Here's how the part is built. I have some questions about the finished solid (model axes, mm). Face numbers are marked on the shaded views. Round coordinates to 2 decimals unless told otherwise and drop trailing zeros. Loops run counter-clockwise (first coordinate to the right, second up) from the corner with the lowest first, then second, coordinate; pieces in that order, holes last. Notation, with made-up numbers: M 17,-21 L 51,-21 A19 cw 51,-11 Z; hole C 61,-5 d9. An arc over 180 degrees is marked long. Use a Markdown table: item, result.
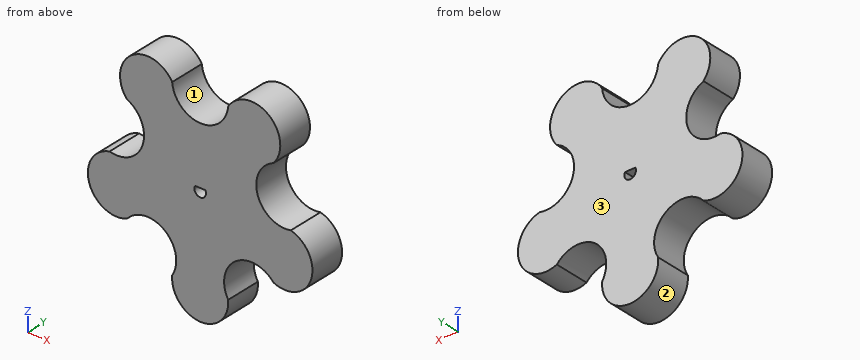
from build123d import *

# Parameters (mm, degrees)
BOSS_EXTRUDE1_DEPTH = 6.35
CUT_EXTRUDE1_DEPTH  = 87.982615074


with BuildPart() as part:
    # Sketch5 → Boss-Extrude1 (new body)
    with BuildSketch(Plane(origin=(0, 0, 0), x_dir=(1, 0, 0), z_dir=(0, 1, 0))):
        with BuildLine():
            ThreePointArc((63.790074828, 30.282665757), (58.727566665, 35.783867727), (53.665058502, 30.282665757))
            ThreePointArc((53.665058502, 30.282665757), (52.307776139, 23.537951339), (45.473748225, 24.331330481))
            ThreePointArc((45.473748225, 24.331330481), (38.677393188, 21.216564002), (42.344946112, 14.701867727))
            ThreePointArc((42.344946112, 14.701867727), (48.340127394, 11.326784114), (45.473748225, 5.072404972))
            ThreePointArc((45.473748225, 5.072404972), (46.335877976, -2.353828549), (53.665058502, -0.878930303))
            ThreePointArc((53.665058502, -0.878930303), (58.727566665, 3.779867727), (63.790074828, -0.878930303))
            ThreePointArc((63.790074828, -0.878930303), (71.119255353, -2.353828549), (71.981385104, 5.072404972))
            ThreePointArc((71.981385104, 5.072404972), (69.115005936, 11.326784114), (75.110187217, 14.701867727))
            ThreePointArc((75.110187217, 14.701867727), (78.777740141, 21.216564002), (71.981385104, 24.331330481))
            ThreePointArc((71.981385104, 24.331330481), (65.14735719, 23.537951339), (63.790074828, 30.282665757))
        make_face()
    extrude(amount=BOSS_EXTRUDE1_DEPTH)

    # Sketch6 → Cut-Extrude1 (cut, through all)
    with BuildSketch(Plane(origin=(0, 0, 0), x_dir=(1, 0, 0), z_dir=(0, 1, 0))):
        with BuildLine():
            Line((57.794311073, 14.225617727), (59.660822257, 14.225617727))
            ThreePointArc((59.660822257, 14.225617727), (58.727566665, 15.749617727), (57.794311073, 14.225617727))
        make_face()
    extrude(amount=CUT_EXTRUDE1_DEPTH, mode=Mode.SUBTRACT)


solid = part.part
1. Imagine slicing it at B-B, the plane x = 69.5. Write out the boundary of the cut face in (y, z).
Answer sheet:
| item | result |
|---|---|
| outline | M 0,-22.76 L 6.35,-22.76 L 6.35,-12.21 L 0,-12.21 Z; M 0,-7.3 L 6.35,-7.3 L 6.35,3.14 L 0,3.14 Z |
2. I need wall thicknesses on probe 1 along X at (y, z) = (5, -23.5); probe 2 along X at (y, z) = (2.5, -31); probe 3 along X at (y, z) = (2.25, -9.5). Which ranges of each line are inside material? Lowest first, please. Write a range as from..to.
Answer sheet:
| item | result |
|---|---|
| probe 1 | 40.2..46.39, 52.25..65.2, 71.07..77.26 |
| probe 2 | 53.66..63.8 |
| probe 3 | 48.58..68.87 |
3. Imagine slicing it at C-C, the plane y = 2.75. Write out the boundary of the cut face in (x, z).
Answer sheet:
| item | result |
|---|---|
| outline | M 42.34,-14.7 A5.08 ccw long 45.47,-24.33 A5.08 cw 53.67,-30.28 A5.08 ccw long 63.79,-30.28 A5.08 cw 71.98,-24.33 A5.08 ccw long 75.11,-14.7 A5.08 cw 71.98,-5.07 A5.08 ccw long 63.79,0.88 A5.08 cw 53.67,0.88 A5.08 ccw long 45.47,-5.07 A5.08 cw Z; hole M 57.79,-14.23 A1.05 ccw long 59.66,-14.23 Z |
4. For pin 1 Ø1.5 at (y, z) = (3.5, -22.5) entering from +X; pin 2 Ø1.5 at (x, y) = (66, 5.5) entering from -Z, each with a flat end and sliding along its axis, tell me the tip position at first contact or that it passes through.
Answer sheet:
| item | result |
|---|---|
| pin 1 | x = 78.57 |
| pin 2 | z = -23.47 |
5. Imagine slicing it at D-D, the plane z = -28. Write out the boundary of the cut face in (x, y).
Answer sheet:
| item | result |
|---|---|
| outline | M 54.39,0 L 63.07,0 L 63.07,6.35 L 54.39,6.35 Z |
6. Imagine slicing it at A-A, the plane z = -3. Write out the boundary of the cut face in (x, y).
Answer sheet:
| item | result |
|---|---|
| outline | M 44.4,0 L 56.02,0 L 56.02,6.35 L 44.4,6.35 Z; M 61.43,0 L 73.06,0 L 73.06,6.35 L 61.43,6.35 Z |
7. We'd pull the mould along X, two halves only. Please class the marked faces 1, 2 and 3: +X half, -X half, draft (parallel to the pull), parting line (faces both ways), or undercut.
Answer sheet:
| item | result |
|---|---|
| face 1 | undercut |
| face 2 | parting line |
| face 3 | draft |
